```python
from build123d import *

# Parameters (mm, degrees)
BOSS_EXTRUDE1_DEPTH      = 7.62
BOSS_EXTRUDE2_DEPTH      = 25.4
BOSS_EXTRUDE2_DEPTH_BACK = 7.62
BOSS_EXTRUDE3_DEPTH      = 7.62


with BuildPart() as part:
    # Sketch1 → Boss-Extrude1 (new body)
    with BuildSketch(Plane.XY):
        Polygon((12.895742644, -26.081168803), (29.034826066, -1.872543671), (16.139083421, 24.208625132), (-12.895742644, 26.081168803), (-29.034826066, 1.872543671), (-16.139083421, -24.208625132), align=None)
        Polygon((9.677238391, -3.016857054), (7.451294044, 6.872305758), (-2.225944347, 9.889162812), (-9.677238391, 3.016857054), (-7.451294044, -6.872305758), (2.225944347, -9.889162812), align=None, mode=Mode.SUBTRACT)
    extrude(amount=-BOSS_EXTRUDE1_DEPTH)

    # Sketch1_3 → Boss-Extrude2 (add, two sides)
    with BuildSketch(Plane.XY) as boss_extrude2_sk:
        Polygon((2.225944347, -9.889162812), (9.677238391, -3.016857054), (7.451294044, 6.872305758), (-2.225944347, 9.889162812), (-9.677238391, 3.016857054), (-7.451294044, -6.872305758), align=None)
        Polygon((5.545838686, -1.911074723), (4.427958602, 3.847299826), (-1.117880084, 5.758374549), (-5.545838686, 1.911074723), (-4.427958602, -3.847299826), (1.117880084, -5.758374549), align=None, mode=Mode.SUBTRACT)
    extrude(amount=BOSS_EXTRUDE2_DEPTH)
    extrude(boss_extrude2_sk.sketch, amount=-BOSS_EXTRUDE2_DEPTH_BACK)

    # Sketch2 → Boss-Extrude3 (add)
    with BuildSketch(Plane(origin=(0, 0, -7.62), x_dir=(-1, 0, 0), z_dir=(0, 0, -1))):
        Polygon((1.117880084, 5.758374549), (-4.427958602, 3.847299826), (-5.545838686, -1.911074723), (-1.117880084, -5.758374549), (4.427958602, -3.847299826), (5.545838686, 1.911074723), align=None)
    extrude(amount=-BOSS_EXTRUDE3_DEPTH)


solid = part.part
```
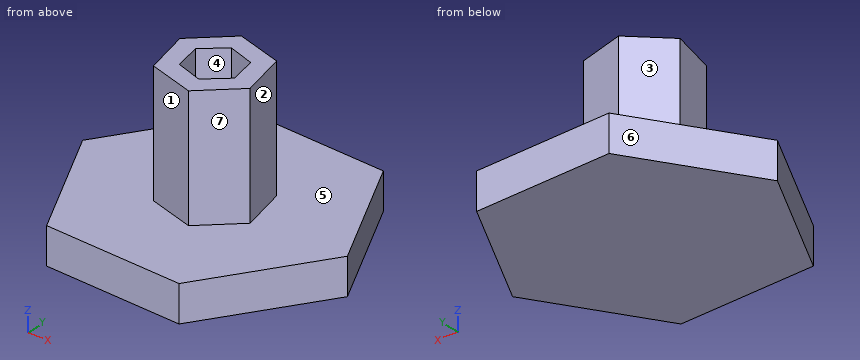
Verification items for the finished model (mm, model axes). Face numbers are marked on the shaded views. A direction names the side the tool comes from. Coordinates: 2 decimals unless noted, no trailing zeros. Loops run counter-clockwise (first coordinate to the right, second up) from the corner with the lowest first, then second, coordinate; pieces in that order, holes last. Notation, with made-up numbers: (62, 72.5) - (101, 72.5) arc R31 ccw to (101, 102.5) - close; hole circle Ø8 at (-10, -14). An arc over 180 degrees is marked (long way). Put each result on its own line as item: value.
Item 1: Section check D-D (y = -9). Enter the section's corners in (x, z).
Conclusion:
outline: (-23.66, -7.62) - (24.28, -7.62) - (24.28, 0) - (3.19, 0) - (3.19, 25.4) - (-0.63, 25.4) - (-0.63, 0) - (-23.66, 0) - close
Item 2: Section check B-B (y = 8). Enter the section's corners in (x, z).
Conclusion:
outline: (-24.95, -7.62) - (24.15, -7.62) - (24.15, 0) - (3.83, 0) - (3.83, 25.4) - (-4.27, 25.4) - (-4.27, 0) - (-24.95, 0) - close
Item 3: Scan lines: line 1 along Z through (x, y) = (-13, 16); line 2 along X through (y, z) = (2, 8); line 3 along Y through (x, z) = (3.5, 21.5). Record each from-to range of solid material in increasing order.
Conclusion:
line 1: z = -7.62 to 0
line 2: x = -9.45 to -5.44, 4.79 to 8.55
line 3: y = -8.71 to -3.69, 4.17 to 8.1
Item 4: Draft check along Y on the marked faces 4, 5, 6 and 7. Enter one of: pulls with the +Y half, pulls with the -Y half, needs draft (parallel to the pull), parting line crosses it, or undercut.
Conclusion:
face 4: undercut
face 5: needs draft
face 6: pulls with the +Y half
face 7: pulls with the -Y half
Item 5: Section check C-C (x = -19). Enter the section's corners in (y, z), then the cut area to 3 significant figures.
Conclusion:
outline: (-18.42, -7.62) - (16.92, -7.62) - (16.92, 0) - (-18.42, 0) - close
area: 269 mm2
Item 6: Gauge pin test, flat ends, axial feed: pin 1 Ø5.5 at (x, y) = (0.5, -1.5) entering from +Z; pin 2 Ø4 at (y, z) = (-8, -0.5) entering from +X. Record the tip position at first contact, or that the pin passes through.
Conclusion:
pin 1: stops at z = 0
pin 2: stops at x = 26.28
Item 7: Section check A-A (z = 13). Enter the section's corners in (x, y).
Conclusion:
outline: (-9.68, 3.02) - (-7.45, -6.87) - (2.23, -9.89) - (9.68, -3.02) - (7.45, 6.87) - (-2.23, 9.89) - close; hole (-5.55, 1.91) - (-4.43, -3.85) - (1.12, -5.76) - (5.55, -1.91) - (4.43, 3.85) - (-1.12, 5.76) - close
Item 8: Set-up check for the marked faces 1, 2 and 3: record each of +Z, -Z, +X, -X, +Y, -Y from which the full face is reachable in a straight line by a thin tool's end or side.
Conclusion:
face 1: +Z, -X, -Y
face 2: +Z, +X, +Y
face 3: +Z, -X, +Y
